Verification items for the finished model (mm, model axes). A direction names the side the tool comes from. Give positions to 0.01 mm unless a question says otherwise; leave off trailing zeros. Order: outer loops, then holes, each group sorted by start corner. A loop starts at its lowest first (then second) coordinate and runs counter-clockwise, first axis right, second up. Notation, with made-up numbers: M 75.25,34.5 L 79.25,34.5 A11 ccw 79.25,44.5 Z; hole C 72.5,-10 d10. An arc over 180 degrees is marked long. Answer as a JSON object with one key per item and string values.
Autodesk Fusion 360 part; units mm, degrees
sketch "Skizze1" plane through (0, 0, 0) normal (0, 0, 1) x (1, 0, 0)
  line L0 (-50, 40) -> (0, 40) construction
  circle A0 centre (-50, 40) radius 3.25
  circle A1 centre (0, 40) radius 3.25
  line L1 (-25, 40) -> (-25, -4) construction
  line L2 (-25, -4) -> (0, -4) construction
  line L3 (0, -4) -> (-50, -4) construction
  circle A2 centre (-50, -4) radius 3.25
  circle A3 centre (0, -4) radius 3.25
  circle A4 centre (-50, 40) radius 6
  circle A5 centre (0, 40) radius 6
  circle A6 centre (0, -4) radius 6
  circle A7 centre (-50, -4) radius 6
  line L4 (-50, -4) -> (0, 40) construction
  line L5 (0, -4) -> (-50, 40) construction
  line L6 (-50, 40) -> (-50, 46) construction
  line L7 (-50, 40) -> (-49.8093, 40.2167) construction
  line L8 (-50, 40) -> (-45.7574, 44.2426) construction
  line L9 (-50, 40) -> (-44, 40) construction
  line L10 (-50, 40) -> (-56, 40) construction
  line L11 (-50, 40) -> (-54.2426, 35.7574) construction
  line L12 (0, -4) -> (6, -4) construction
  line L13 (0, -4) -> (4.2426, 0.2426) construction
  line L14 (0, -4) -> (6, -4) construction
  line L15 (0, -4) -> (0, -10) construction
  line L16 (0, -4) -> (-4.2426, -8.2426) construction
  line L17 (-4.2426, -8.2426) -> (-54.2426, 35.7574)
  line L18 (4.2426, 0.2426) -> (-45.7574, 44.2426)
  line L19 (0, 40) -> (0, 46) construction
  line L20 (0, 40) -> (-4.2426, 44.2426) construction
  line L21 (0, 40) -> (4.2426, 35.7574) construction
  line L22 (0, 40) -> (6, 40) construction
  line L23 (-50, -4) -> (-45.7574, -8.2426) construction
  line L24 (-50, -4) -> (-44, -4) construction
  line L25 (-50, -4) -> (-54.2426, 0.2426) construction
  line L26 (-50, -4) -> (-44, -4) construction
  line L27 (-54.2426, 0.2426) -> (-4.2426, 44.2426)
  line L28 (4.2426, 35.7574) -> (-45.7574, -8.2426)
  line L29 (-3.2166, 6.8068) -> (-3.2166, 29.1932)
  line L30 (-40.3073, 12.5057) -> (-40.3073, 23.4943)
  line L31 (-20.7574, 6.2903) -> (-29.2426, 6.2903)
  line L32 (-20.7574, 29.7097) -> (-29.2426, 29.7097)
  dimension "d2" = 6.5
  dimension "d3" = 6.5
  dimension "d4" = 6.5
  dimension "d5" = 6.5
  dimension "d6" = 12
  dimension "d7" = 12
  dimension "d8" = 12
  dimension "d9" = 45
  dimension "d10" = 135
  dimension "d11" = 6
  dimension "d12" = 45
  dimension "d13" = 135
  dimension "d14" = 135
  dimension "d15" = 45
  dimension "d16" = 6
  dimension "d17" = 45
  dimension "d18" = 135
extrude "Extrusion1" add sketch "Skizze1" along normal blind 10 contours A4 L17 | A4 L17 L18 L27 | A5 L18 L27 L28 | L17 L18 L27 L28 | A7 L17 L27 L28 | A6 L17 L18 L28 | A5 L28 | A7 L27 | A6 L18 picked at (-55.035, 39.3919) picked at (-3.2811, 43.8676) picked at (-46.7227, -7.8704) picked at (-3.2811, -7.8676)
extrude "Extrusion2" add sketch "Skizze1" along normal blind 10 contours L18 L27 L32 | L17 L27 L30 | L18 L28 L29 | L17 L28 L31
sketch "Skizze2" plane through (0, 0, 10) normal (0, 0, 1) x (-1, 0, 0)
  circle A0 centre (0, -40) radius 3.25
  circle A1 centre (50, 4) radius 3.25
  circle A2 centre (50, -40) radius 3.25
  circle A3 centre (0, 4) radius 3.25
  line L0 (29.2426, -29.7097) -> (45.7574, -44.2426)
  arc A4 (45.7574, -44.2426) -> (54.2426, -35.7574) centre (50, -40) ccw
  line L1 (54.2426, -35.7574) -> (40.3073, -23.4943)
  line L2 (40.3073, -23.4943) -> (40.3073, -12.5057)
  line L3 (40.3073, -12.5057) -> (54.2426, -0.2426)
  arc A5 (54.2426, -0.2426) -> (45.7574, 8.2426) centre (50, 4) ccw
  line L4 (45.7574, 8.2426) -> (29.2426, -6.2903)
  line L5 (29.2426, -6.2903) -> (20.7574, -6.2903)
  line L6 (20.7574, -6.2903) -> (4.2426, 8.2426)
  arc A6 (4.2426, 8.2426) -> (-4.2426, -0.2426) centre (0, 4) ccw
  line L7 (-4.2426, -0.2426) -> (3.2166, -6.8068)
  line L8 (3.2166, -6.8068) -> (3.2166, -29.1932)
  line L9 (3.2166, -29.1932) -> (-4.2426, -35.7574)
  arc A7 (-4.2426, -35.7574) -> (4.2426, -44.2426) centre (0, -40) ccw
  line L10 (4.2426, -44.2426) -> (20.7574, -29.7097)
  line L11 (20.7574, -29.7097) -> (29.2426, -29.7097)
  line L12 (5.2166, -8.2903) -> (38.3073, -8.2903) construction
  line L13 (38.3073, -8.2903) -> (38.3073, -27.7097) construction
  line L14 (38.3073, -27.7097) -> (5.2166, -27.7097) construction
  line L15 (5.2166, -27.7097) -> (5.2166, -8.2903) construction
  line L16 (3.2166, -6.8068) -> (3.2166, -29.1932) construction
  line L17 (5.2166, -8.2903) -> (38.3073, -8.2903)
  line L18 (38.3073, -8.2903) -> (38.3073, -27.7097)
  line L19 (38.3073, -27.7097) -> (5.2166, -27.7097)
  line L20 (5.2166, -27.7097) -> (5.2166, -8.2903)
  dimension "d24" = 2
  dimension "d25" = 2
  dimension "d26" = 2
  dimension "d27" = 2
extrude "Extrusion3" cut sketch "Skizze2" against normal blind 8 contours L17 L18 L19 L20
sketch "Skizze3" plane through (0, 0, 10) normal (0, 0, 1) x (-1, 0, 0)
  line L0 (38.3073, -8.2903) -> (38.3073, -27.7097)
  line L1 (38.3073, -27.7097) -> (5.2166, -27.7097)
  line L2 (5.2166, -27.7097) -> (5.2166, -8.2903)
  line L3 (5.2166, -8.2903) -> (38.3073, -8.2903)
  circle A0 centre (0, -40) radius 3.25
  circle A1 centre (50, 4) radius 3.25
  circle A2 centre (50, -40) radius 3.25
  circle A3 centre (0, 4) radius 3.25
  line L4 (29.2426, -29.7097) -> (45.7574, -44.2426)
  arc A4 (45.7574, -44.2426) -> (54.2426, -35.7574) centre (50, -40) ccw
  line L5 (54.2426, -35.7574) -> (40.3073, -23.4943)
  line L6 (40.3073, -23.4943) -> (40.3073, -12.5057)
  line L7 (40.3073, -12.5057) -> (54.2426, -0.2426)
  arc A5 (54.2426, -0.2426) -> (45.7574, 8.2426) centre (50, 4) ccw
  line L8 (45.7574, 8.2426) -> (29.2426, -6.2903)
  line L9 (29.2426, -6.2903) -> (20.7574, -6.2903)
  line L10 (20.7574, -6.2903) -> (4.2426, 8.2426)
  arc A6 (4.2426, 8.2426) -> (-4.2426, -0.2426) centre (0, 4) ccw
  line L11 (-4.2426, -0.2426) -> (3.2166, -6.8068)
  line L12 (3.2166, -6.8068) -> (3.2166, -29.1932)
  line L13 (3.2166, -29.1932) -> (-4.2426, -35.7574)
  arc A7 (-4.2426, -35.7574) -> (4.2426, -44.2426) centre (0, -40) ccw
  line L14 (4.2426, -44.2426) -> (20.7574, -29.7097)
  line L15 (20.7574, -29.7097) -> (29.2426, -29.7097)
  line L16 (48.8732, -36.9516) -> (38.0802, -26.1585)
  line L17 (48.8732, -36.9516) -> (64.1369, -36.9516) construction
  line L18 (46.8537, -39.1856) -> (34.6878, -27.7097)
  line L19 (48.8732, -36.9516) -> (46.8537, -39.1856)
  line L20 (38.0802, -26.1585) -> (34.6878, -27.7097)
  line L21 (1.4355, -37.0842) -> (7.4315, -27.7097)
  line L22 (11.379, -27.7097) -> (11.379, -27.9297)
  line L23 (11.379, -27.9297) -> (2.8213, -38.3867)
  line L24 (11.379, -27.7097) -> (7.4315, -27.7097)
  line L25 (2.8213, -38.3867) -> (1.4355, -37.0842)
  line L26 (1.0685, 0.9307) -> (9.1829, -8.2903)
  line L27 (2.9716, 2.684) -> (12.3168, -8.2903)
  line L28 (47.853, 1.5602) -> (47.9543, 1.6753)
  line L29 (47.9543, 1.6753) -> (38.3073, -9.8074)
  line L30 (46.9218, 5.0426) -> (46.0785, 2.5527)
  line L31 (46.0785, 2.5527) -> (36.9689, -8.2903)
  line L32 (38.3073, -9.8074) -> (36.9689, -8.2903)
  line L33 (46.9218, 5.0426) -> (46.9218, 4.5082)
  line L34 (46.9218, 4.5082) -> (47.853, 1.5602)
  line L35 (2.9716, 2.684) -> (1.0685, 0.9307)
  line L36 (12.3168, -8.2903) -> (9.1829, -8.2903)
  line L37 (9.1829, -8.2903) -> (12.3168, -8.2903)
  dimension "d30" = 135
extrude "Extrusion4" cut sketch "Skizze3" against normal blind 6 contours L0 L3 A1 L29 L30 L31 | L0 L1 A2 L16 L18 | L3 A3 L26 L27 L36 L37 | L1 A0 L21 L22 L23 L24
extrude "Extrusion5" add sketch "Skizze3" against normal blind 2.5 contours L0 L3 A1 L29 L30 L31 | L0 L1 A2 L16 L18 | L3 A3 L26 L27 L36 L37 | L1 A0 L21 L22 L23 L24
sketch "Skizze4" plane through (0, 0, 10) normal (0, 0, 1) x (-1, 0, 0)
  circle A0 centre (39, -29.5) radius 1.5
  circle A1 centre (7, -30) radius 1.5
  circle A2 centre (40, -8) radius 1.5
  circle A3 centre (6, -6) radius 1.5
  dimension "d35" = 3
  dimension "d36" = 3
  dimension "d37" = 3
  dimension "d38" = 3
extrude "Extrusion6" add sketch "Skizze4" along normal blind 5
sketch "Skizze5" plane through (0, 0, 15) normal (0, 0, 1) x (-1, 0, 0)
  circle A0 centre (40, -8) radius 1.5
  line L0 (4, -4) -> (42, -4)
  line L1 (42, -4) -> (42, -32)
  line L2 (42, -32) -> (4, -32)
  line L3 (4, -32) -> (4, -4)
extrude "Extrusion7" add sketch "Skizze5" along normal blind 1 contours A0 | L0 L1 L2 L3
sketch "Skizze6" plane through (0, 0, 16) normal (0, 0, 1) x (-1, 0, 0)
  line L0 (4, -32) -> (42, -32)
  line L1 (42, -32) -> (42, -4)
  line L2 (42, -4) -> (4, -4)
  line L3 (4, -4) -> (4, -32)
  line L4 (42, -27) -> (10, -27)
  line L5 (10, -27) -> (10, -9)
  line L6 (10, -9) -> (42, -9)
  line L7 (42, -9) -> (42, -4)
  line L8 (4, -4) -> (4, -32)
  line L9 (42, -32) -> (42, -27)
  dimension "d43" = 5
  dimension "d44" = 5
  dimension "d45" = 6
extrude "Extrusion8" add sketch "Skizze6" along normal blind 5 contours L0 L1 L2 L3 L4 L5 L6 L7 L8 L9
sketch "Skizze7" plane through (0, 0, 16) normal (0, 0, 1) x (-1, 0, 0)
  line L0 (42, -9) -> (10, -9)
  line L1 (10, -9) -> (10, -27)
  line L2 (10, -27) -> (42, -27)
  line L3 (42, -27) -> (42, -9)
  line L4 (42, -23) -> (39, -23)
  line L5 (39, -23) -> (39, -13)
  line L6 (39, -13) -> (42, -13)
  line L7 (42, -23) -> (42, -13)
extrude "Extrusion9" cut sketch "Skizze7" against normal blind 1 contours L3 L4 L5 L6 L7
sketch "Skizze8" plane through (0, 27, 0) normal (0, -1, 0) x (1, 0, 0)
  line L0 (-42, 16) -> (-10, 16)
  line L1 (-10, 16) -> (-10, 21)
  line L2 (-10, 21) -> (-42, 21)
  line L3 (-42, 21) -> (-42, 16)
  line L4 (-42, 19) -> (-10, 19)
extrude "Extrusion10" add sketch "Skizze8" along normal blind 2 contours L1 L2 L3 L4
sketch "Skizze9" plane through (0, 9, 0) normal (0, 1, 0) x (-1, 0, 0)
  line L0 (10, 16) -> (42, 16)
  line L1 (42, 16) -> (42, 21)
  line L2 (42, 21) -> (10, 21)
  line L3 (10, 21) -> (10, 16)
  line L4 (10, 19) -> (42, 19)
extrude "Extrusion11" add sketch "Skizze9" along normal blind 2 contours L1 L2 L3 L4
sketch "Skizze10" plane through (-10, 0, 0) normal (-1, 0, 0) x (0, -1, 0)
  line L0 (-11, 19) -> (-11, 21)
  line L1 (-11, 21) -> (-25, 21)
  line L2 (-25, 21) -> (-25, 19)
  line L3 (-25, 19) -> (-27, 19)
  line L4 (-27, 19) -> (-27, 16)
  line L5 (-27, 16) -> (-9, 16)
  line L6 (-9, 16) -> (-9, 19)
  line L7 (-9, 19) -> (-11, 19)
  line L8 (-25, 19) -> (-11, 19)
extrude "Extrusion12" add sketch "Skizze10" along normal blind 5 contours L0 L1 L2 L8
Q1. Section check A-A on x = -43.5. Record the cut outline in (y, z), then the cut area to 3 significant figures.
Resolved:
{"outline": "M -6.26,0 L 9.7,0 L 9.7,10 L -6.26,10 Z; M 26.3,0 L 42.26,0 L 42.26,10 L 26.3,10 Z; hole M 0.52,4 L 3.63,4 L 3.63,7.5 L 0.52,7.5 Z; hole M 31.58,4 L 36.02,4 L 36.02,7.5 L 31.58,7.5 Z", "area": "293 mm²"}
Q2. Section check B-B on y = 33.5. Record the cut outline in (x, z).
Resolved:
{"outline": "M -51.68,0 L -33.55,0 L -33.55,10 L -51.68,10 Z; M -16.45,0 L 1.68,0 L 1.68,10 L -16.45,10 Z; hole M -45.42,4 L -40.83,4 L -40.83,7.5 L -45.42,7.5 Z; hole M -6.82,4 L -3.73,4 L -3.73,7.5 L -6.82,7.5 Z"}
Q3. Material ranges on L1, parallel to Y at x = -21.5, z = 20.25; L2, parallel to X at y = 40, z = 1.5; L3, parallel to Y at x = 2.5, z = 9.5, recorded low to high.
Resolved:
{"L1": "y = 4 to 11, 25 to 32", "L2": "x = -56 to -53.25, -46.75 to -40.94, -9.06 to -3.25, 3.25 to 6", "L3": "y = -9.45 to -6.08, -1.92 to 1.78, 34.22 to 37.92, 42.08 to 45.45"}
Q4. Release check for a two-part mould opening along Z. For faces 6 (the face through (-37.38, -0.87, 4.93)), 7 (the face through (-37.89, 30.51, 12.46)) record: +Z half, -Z half, draft (parallel to the pull), parting line (faces both ways), or undercut.
Resolved:
{"face 6": "draft", "face 7": "undercut"}
Q5. Tool access check on faces 1 (the face through (-43.148, 4.045, 5.774)), 2 (the face through (1.75, -6.74, 4.93)), 3 (the face through (-26, 27, 17)), 4 (the face through (-42, 29, 18)), 5 (the face through (-23, 4, 18)). Record the directions out of +Z, -Z, +X, -X, +Y, -Y that give a thin tool (end or side, any length) a straight path to the whole face; none if there is none.
Resolved:
{"face 1": "none", "face 2": "+Z, -Z", "face 3": "-X", "face 4": "+Z, -X, +Y, -Y", "face 5": "+Z, +X, -X, -Y"}
Q6. Section check D-D on x = -35.5. Record the cut outline in (y, z), then the cut area to 3 significant figures.
Resolved:
{"outline": "M 0.78,0 L 35.22,0 L 35.22,10 L 27.71,10 L 27.71,7.5 L 28.48,7.5 L 28.48,4 L 27.71,4 L 27.71,2 L 8.29,2 L 8.29,10 L 0.78,10 Z; M 4,15 L 32,15 L 32,21 L 25,21 L 25,19 L 27,19 L 27,16 L 9,16 L 9,19 L 11,19 L 11,21 L 4,21 Z", "area": "272 mm²"}
Q7. Section check C-C on z = 18.25. Record the cut outline in (x, y).
Resolved:
{"outline": "M -42,4 L -4,4 L -4,32 L -42,32 L -42,27 L -10,27 L -10,9 L -42,9 Z"}
Q8. Gauge pin test, flat ends, axial feed: pin 1 Ø2.5 at (y, z) = (22.5, 6.5) entering from +X; pin 2 Ø1.5 at (x, y) = (-33, 12) entering from +Z; pin 3 Ø6.5 at (y, z) = (6.5, 18.5) entering from -X; pin 4 Ø14.5 at (x, y) = (-29.5, 13.5) entering from -Z. Record the tip position at first contact, or that the pin passes through.
Resolved:
{"pin 1": "stops at x = -3.22", "pin 2": "stops at z = 16", "pin 3": "stops at x = -42", "pin 4": "stops at z = 0"}
